```python
from build123d import *

# Parameters (mm, degrees)
SKETCH_1_R             = 5.75
EXTRUDE_1_DEPTH        = 50
HOLE_WIZARD_M5_1_D     = 4.2
HOLE_WIZARD_M5_1_DEPTH = 12.4
HOLE_WIZARD_M5_1_TIP   = 1.2618073


with BuildPart() as part:
    # 草图1 → 凸台-拉伸1 (new body)
    with BuildSketch(Plane.XY):
        Polygon((6.273575685, -7.78731328), (9.88079897, 1.539419276), (3.607223285, 9.326732556), (-6.273575685, 7.78731328), (-9.88079897, -1.539419276), (-3.607223285, -9.326732556), align=None)
        Circle(SKETCH_1_R, mode=Mode.SUBTRACT)
    extrude(amount=EXTRUDE_1_DEPTH)

    # M5 螺纹孔1
    with Locations(Plane(origin=(-6.744011128, -5.433075916, 0), x_dir=(0, 0, 1), z_dir=(-0.7787313279896286, -0.6273575685424616, 0))):
        with Locations((9.322042098, 0)):
            Hole(HOLE_WIZARD_M5_1_D / 2, depth=HOLE_WIZARD_M5_1_DEPTH)
            with Locations((0, 0, -(HOLE_WIZARD_M5_1_DEPTH + HOLE_WIZARD_M5_1_TIP / 2))):  # 118° drill point
                Cone(0, HOLE_WIZARD_M5_1_D / 2, HOLE_WIZARD_M5_1_TIP, mode=Mode.SUBTRACT)


solid = part.part
```
Design review of the part built by this model. Coordinates are the model's own, in mm. Give positions to 0.01 mm unless a question says otherwise; leave off trailing zeros. Write each loop counter-clockwise with the first axis right and the second up, starting at its lowest first coordinate (ties: lowest second). Pieces come first, ordered by that corner, then holes. Notation, with made-up numbers: (-9.75, 86.25) - (14.25, 86.25) arc R20 ccw to (14.25, 117.25) - close; hole circle Ø11 at (-27, -6). An arc over 180 degrees is marked (long way). Return JSON: item names as keys, results as strings. Group by question number.
(1) We need section B-B, the plane x = -1.25. Give the boundary of the cut face in (y, z), then the cut area to 3 significant figures.
(2) We need section C-C, the plane y = 0. Give the boundary of the cut face in (x, z).
(3) Insertion check: pin 1 (5 mm diameter, centred on x = -4, z = 12, fed in from -Y); pin 2 (6 mm diameter, centred on x = 3.5, z = 6, fed in from +Y); pin 3 (8 mm diameter, centred on x = -3, z = 8.5, fed in from +Y). Each pin has a flat end and moves straight along its axis. Give the tip position at first contact, or say it passes through.
(4) We need section D-D, the plane y = -4.75. Give the number of separate pieces and of enclosed holes in the cut face, then the cut area to 3 significant figures.
(5) To check wall thickness, follow probe 1 along Y at (x, z) = (0, 35.5); probe 2 along Y at (x, z) = (-1.25, 7); probe 3 along Z at (x, y) = (-5, -3.25). State the ranges of each line that lie inside material, in increasing order.
(6) We need section A-A, the plane z = 5. Give the boundary of the cut face in (x, y), then the cut area to 3 significant figures.
(7) Mouldability with a two-part tool opening along Y and no side actions: class faces 1 (the flat face through (-6.788, -5.379, 24.65)), 2 (the cylindrical face through (5.484, 1.727, 24.65)), 3 (the cylindrical face through (-4.933, -5.007, 7.382)), 4 (the flat face through (-8.05, 3.19, 24.65)) as +Y half, -Y half, draft (parallel to the pull), parting line (faces both ways), or undercut.
Reported:
{
 "1": {"outline": "(-8.96, 0) - (-5.61, 0) - (-5.61, 50) - (-8.96, 50) - close; (5.61, 0) - (8.57, 0) - (8.57, 50) - (5.61, 50) - close", "area": "315 mm2"},
 "2": {"outline": "(-9.29, 0) - (-5.75, 0) - (-5.75, 50) - (-9.29, 50) - close; (5.75, 0) - (9.29, 0) - (9.29, 50) - (5.75, 50) - close"},
 "3": {"pin 1": "stops at y = -9.33", "pin 2": "stops at y = 9.33", "pin 3": "stops at y = 8.92"},
 "4": {"separate pieces": "3", "enclosed holes": "0", "area": "398 mm2"},
 "5": {"probe 1": "y = -8.76 to -5.75, 5.75 to 8.76", "probe 2": "y = -8.96 to -5.61, 5.61 to 8.57", "probe 3": "z = 0 to 7.31, 11.33 to 50"},
 "6": {"outline": "(-9.88, -1.54) - (-3.61, -9.33) - (6.27, -7.79) - (9.88, 1.54) - (3.61, 9.33) - (-6.27, 7.79) - close; hole circle Ø11.5 at (0, 0)", "area": "156 mm2"},
 "7": {"face 1": "-Y half", "face 2": "undercut", "face 3": "undercut", "face 4": "+Y half"}
}
